Here's how the part is built. I have some questions about the finished solid (model axes, mm). Face numbers are marked on the shaded views. A direction names the side the tool comes from. Round coordinates to 2 decimals unless told otherwise and drop trailing zeros. Write each loop counter-clockwise with the first axis right and the second up, starting at its lowest first coordinate (ties: lowest second). Pieces come first, ordered by that corner, then holes. Notation, with made-up numbers: (-23.5, 42) -> (-10.5, 42) arc R22 cw to (-10.5, 73) -> close; hole circle Ø1 at (40, 83.25). An arc over 180 degrees is marked (long way). Put each result on its own line as item: value. Start each with the question number.
1) Which directions (+Z, -Z, +X, -X, +Y, -Y) give clear straight access to the entire face, cutting with the end or side of a thin tool? Please do the marked faces 1 and 2.
2) Will these pins go through, and if not, where does the flat tip stop? P1, Ø8, axis at x = -35.5, y = 19.5, coming from the -Z side; P2, Ø12, axis at y = -4, z = -53, coming from the -X side; P3, Ø10, axis at y = -4.5, z = 35, coming from the -X side.
3) I want a section at A-A, the plane y = -14.5. List the corners of the cut face in (x, z) for me, then the cut area to 3 significant figures.
4) If I drill on line 1 along Y through (x, z) = (4, 7.5); line 2 along Y through (x, z) = (-55, 20); line 3 along X through (y, z) = (3.5, 44.5), over which ranges is the centre line in solid material (lowest first)? Write a range as [from, to].
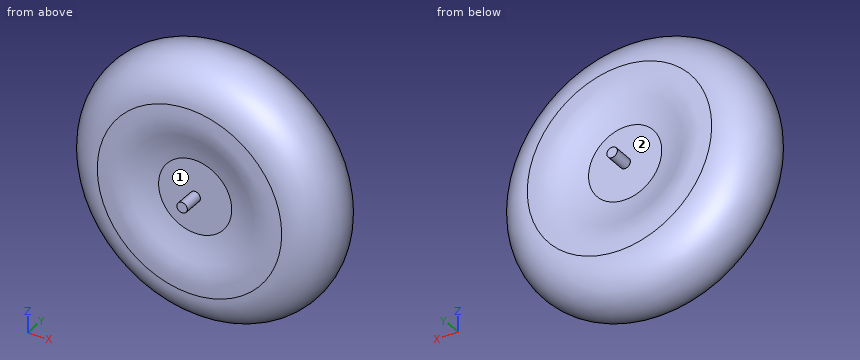
from build123d import *

# Parameters (mm, degrees)
F2_R     = 3
F3_DEPTH = 29


with BuildPart() as f1:
    # F0 (on Top) → F1 (revolve)
    with BuildSketch(Plane.XY):
        with BuildLine():
            Line((-3, 0), (-3, 17.4995933901))
            Line((-3, 17.4995933901), (-21, 17.4995933901))
            add(Edge.make_bspline(
                [(-52.9111102223, 22.5), (-49.0063974427, 22.770887551), (-41.4137818802, 23.2581714642), (-31.7984179158, 19.6037849598), (-24.6587238594, 18.0655321125), (-21, 17.4995933901)],
                knots=[0, 0, 0, 0, 0.3420035898, 0.664256839, 1, 1, 1, 1], degree=3))
            ThreePointArc((-52.9111102223, 22.5), (-75.1510886965, 0), (-52.9111102223, -22.5))
            add(Edge.make_bspline(
                [(-52.9111102223, -22.5), (-49.0063974427, -22.770887551), (-41.4137818802, -23.2581714642), (-31.7984179158, -19.6037849598), (-24.6587238594, -18.0655321125), (-21, -17.4995933901)],
                knots=[0, 0, 0, 0, 0.3420035898, 0.664256839, 1, 1, 1, 1], degree=3))
            Line((-21, -17.4995933901), (-3, -17.4995933901))
            Line((-3, -17.4995933901), (-3, 0))
        make_face()
    revolve(axis=Axis((0, 13.3384466171, 0), (0, 1, 0)))

    # F2 (on Front) → F3 (join, symmetric)
    with BuildSketch(Plane.XZ):
        Circle(F2_R)
    extrude(amount=F3_DEPTH, both=True)


solid = f1.part
Findings:
1. face 1: -Y
1. face 2: +Y
2. P1: stops at z = -59.69
2. P2: stops at x = -58.32
2. P3: stops at x = -68.58
3. outline: circle Ø139.71 at (0, 0)
3. area: 15,300 mm2
4. line 1: y = [-17.5, 17.5]
4. line 2: y = [-21.72, 21.72]
4. line 3: x = [-60.22, 60.22]
